Job drawing, mm, ordinate dimensions from the low corner. One solid piece. A direction names the side the tool comes from. Give positions to 0.01 mm unless a question says otherwise; leave off trailing zeros. Order: outer loops, then holes, each group sorted by start corner. A loop starts at its lowest first (then second) coordinate and runs counter-clockwise, first axis right, second up.
1. Mould opens along Y. For the marked faces 3, 4 and 5 say: +Y half, -Y half, draft (parallel to the pull), parting line (faces both ways), or undercut.
2. Which spindle directions (+Z, -Z, +X, -X, +Y, -Y) get a long thin tool onto all of the face, cutting with end or side? Do the marked faces 1 and 2. Say none if no direction does.
3. Slice it at C-C on y = 12.75. List the corners of the cut face in (x, z) (1 decimal).
4. Drop flat-ended pins along their axis: pin 1 Ø8.5 at (x, y) = (8.001, 8.001) entering from +Z; pin 2 Ø1 at (y, z) = (11.5, 4.5) entering from +X. Give the stop position or say it passes through.
5. Slice it at B-B on y = 8.5. List the corners of the cut face in (x, z) (1 decimal).
6. Slice it at D-D on x = 1.5. List the corners of the cut face in (y, z) (1 decimal).
7. Probe line 1 (Z direction, x = 6.5, y = 1.25); line 2 (X direction, y = 11.5, z = 4.15) (1 decimal); line 3 (Y direction, x = 5.75, z = 3.05) (1 decimal). List the from-to ranges inside material, lowest first.
8. Slice it at A-A on x = 9.75. List the corners of the cut face in (y, z).
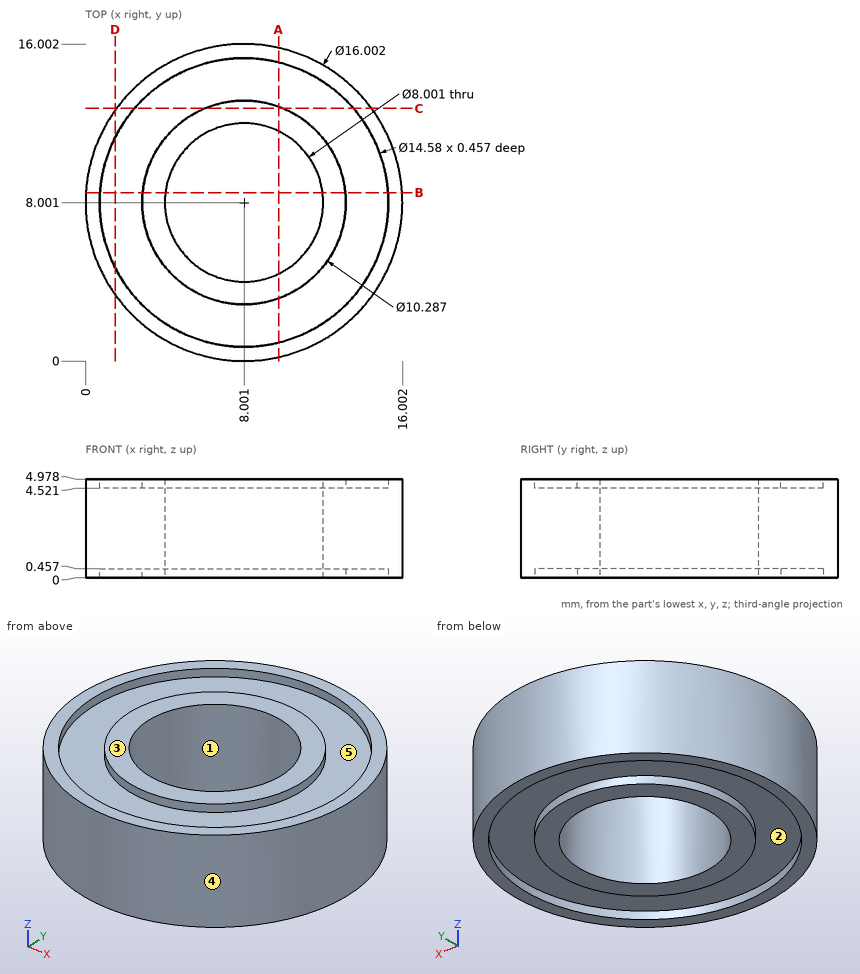
Data:
1. face 3: draft
1. face 4: parting line
1. face 5: undercut
2. face 1: +Z, -Z
2. face 2: -Z
3. outline: (1.6, 0) - (2.5, 0) - (2.5, 0.5) - (6, 0.5) - (6, 0) - (10, 0) - (10, 0.5) - (13.5, 0.5) - (13.5, 0) - (14.4, 0) - (14.4, 5) - (13.5, 5) - (13.5, 4.5) - (10, 4.5) - (10, 5) - (6, 5) - (6, 4.5) - (2.5, 4.5) - (2.5, 5) - (1.6, 5) - close
4. pin 1: stops at z = 4.98
4. pin 2: stops at x = 15.42
5. outline: (0, 0) - (0.7, 0) - (0.7, 0.5) - (2.9, 0.5) - (2.9, 0) - (4, 0) - (4, 5) - (2.9, 5) - (2.9, 4.5) - (0.7, 4.5) - (0.7, 5) - (0, 5) - close; (12, 0) - (13.1, 0) - (13.1, 0.5) - (15.3, 0.5) - (15.3, 0) - (16, 0) - (16, 5) - (15.3, 5) - (15.3, 4.5) - (13.1, 4.5) - (13.1, 5) - (12, 5) - close
6. outline: (3.3, 0) - (4.7, 0) - (4.7, 0.5) - (11.3, 0.5) - (11.3, 0) - (12.7, 0) - (12.7, 5) - (11.3, 5) - (11.3, 4.5) - (4.7, 4.5) - (4.7, 5) - (3.3, 5) - close
7. line 1: z = 0.46 to 4.52
7. line 2: x = 0.8 to 6.1, 9.9 to 15.2
7. line 3: y = 0.3 to 4.7, 11.3 to 15.7
8. outline: (0.19, 0) - (0.92, 0) - (0.92, 0.46) - (3.16, 0.46) - (3.16, 0) - (4.4, 0) - (4.4, 4.98) - (3.16, 4.98) - (3.16, 4.52) - (0.92, 4.52) - (0.92, 4.98) - (0.19, 4.98) - close; (11.6, 0) - (12.84, 0) - (12.84, 0.46) - (15.08, 0.46) - (15.08, 0) - (15.81, 0) - (15.81, 4.98) - (15.08, 4.98) - (15.08, 4.52) - (12.84, 4.52) - (12.84, 4.98) - (11.6, 4.98) - close
